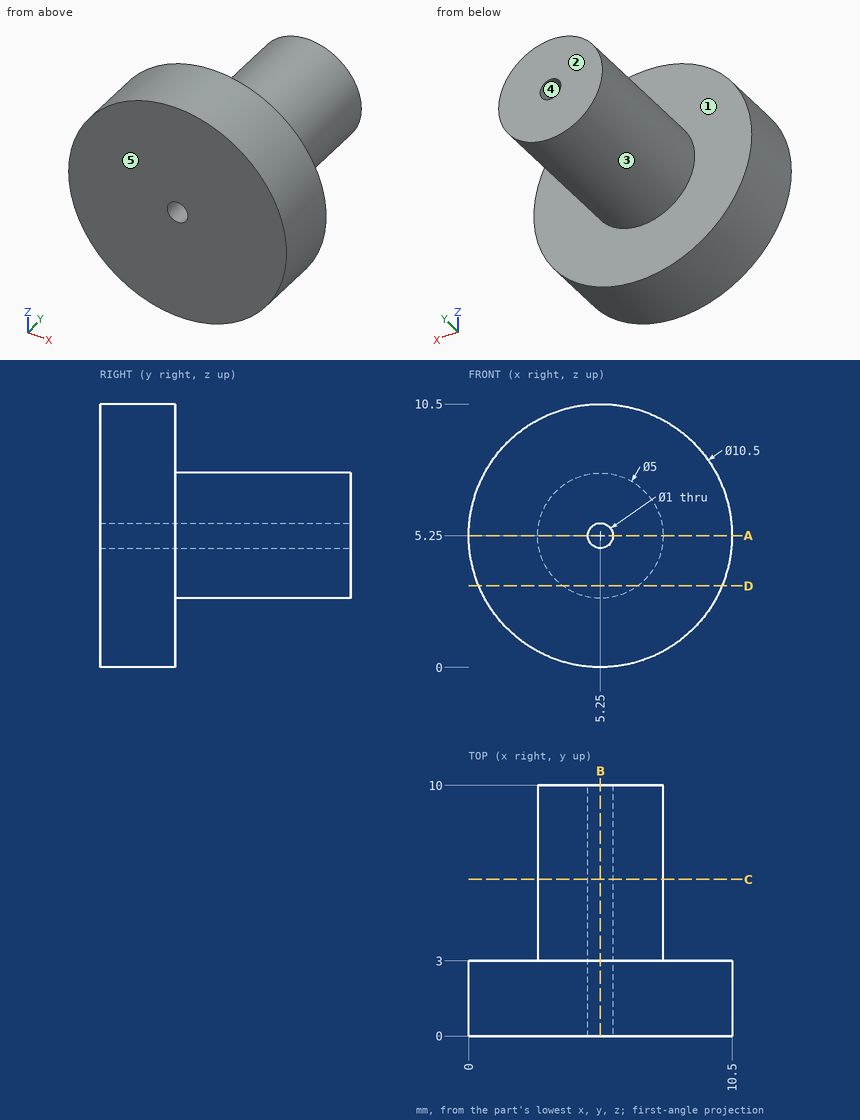
Drawing for the job (mm, zero at the part's lowest x, y, z). A direction names the side the tool comes from. Give positions to 0.01 mm unless a question says otherwise; leave off trailing zeros. Loops run counter-clockwise (first coordinate to the right, second up) from the corner with the lowest first, then second, coordinate; pieces in that order, holes last. Notation, with made-up numbers: (73, 2.5) - (110, 2.5) arc R19 cw to (110, 36.5) - close; hole circle Ø7 at (-0.75, 22.5). An arc over 180 degrees is marked (long way). Write item = value, one per line. Start each with the question number.
1) Pull direction Z, two halves, no side cores. Call the marked faces 3, 4 and 5: +Z half, -Z half, draft (parallel to the pull), parting line (faces both ways), or undercut.
2) Probe probe 1 along Z at (x, y) = (5.25, 7.25); probe 2 along Z at (x, y) = (5.25, 2.25). List the from-to ranges inside material, lowest first. Write a range as from..to.
3) Band-saw the part on D-D on z = 3.25. Give the cut face in (x, y).
4) Band-saw the part on A-A on z = 5.25. Give the cut face in (x, y).
5) Band-saw the part on C-C on y = 6.25. Give the cut face in (x, z), plus the area to 3 significant figures.
6) Tool access for the marked faces 1 and 2: list every direction of +Z, -Z, +X, -X, +Y, -Y with a clear straight run to the whole face (end or side of a thin tool).
7) Band-saw the part on B-B on x = 5.25. Give the cut face in (y, z).
Final values:
q1.face_3 = parting line
q1.face_4 = undercut
q1.face_5 = draft
q2.probe_1 = 2.75..4.75, 5.75..7.75
q2.probe_2 = 0..4.75, 5.75..10.5
q3.outline = (0.4, 0) - (10.1, 0) - (10.1, 3) - (6.75, 3) - (6.75, 10) - (3.75, 10) - (3.75, 3) - (0.4, 3) - close
q4.outline = (0, 0) - (4.75, 0) - (4.75, 10) - (2.75, 10) - (2.75, 3) - (0, 3) - close; (5.75, 0) - (10.5, 0) - (10.5, 3) - (7.75, 3) - (7.75, 10) - (5.75, 10) - close
q5.outline = circle Ø5 at (5.25, 5.25); hole circle Ø1 at (5.25, 5.25)
q5.area = 18.8 mm²
q6.face_1 = +Y
q6.face_2 = +Z, -Z, +X, -X, +Y
q7.outline = (0, 0) - (3, 0) - (3, 2.75) - (10, 2.75) - (10, 4.75) - (0, 4.75) - close; (0, 5.75) - (10, 5.75) - (10, 7.75) - (3, 7.75) - (3, 10.5) - (0, 10.5) - close
